```python
from build123d import *

# Parameters (mm, degrees)
SKETCH1_R              = 17.6
BOSS_EXTRUDE1_DEPTH    = 56.8
BOSS_EXTRUDE2_DEPTH    = 4
SKETCH4_R              = 4
SKETCH4_R_2            = 1.5
CUT_EXTRUDE1_DEPTH     = 4
BOSS_EXTRUDE3_DEPTH    = 16
CUT_EXTRUDE2_START     = -14
CUT_EXTRUDE2_OUTLINE_R = 1.45
CUT_EXTRUDE2_DEPTH     = 14
CUT_EXTRUDE3_DEPTH     = 33


# Read off the part's stored shape, not the designer's step: Cut-Extrude2
with BuildPart() as part:
    # Sketch1 → Boss-Extrude1 (new body)
    with BuildSketch(Plane(origin=(0, 0, 0), x_dir=(1, 0, 0), z_dir=(0, 1, 0))):
        with BuildLine():
            Line((-14, -30.7), (-10.2, -30.7))
            ThreePointArc((-10.2, -30.7), (0, -20.5), (10.2, -30.7))
            Line((10.2, -30.7), (14, -30.7))
            add(Edge.make_bspline(
                [(22.4, 0), (22.107939007, -9.890498416), (16.256040946, -13.947885017), (11.388120446, -21.994772931), (14.153535086, -27.339514928), (14, -30.7)],
                knots=[0, 0, 0, 0, 0.589197799, 0.689197799, 1, 1, 1, 1], degree=3))
            ThreePointArc((22.4, 0), (0, 22.4), (-22.4, 0))
            add(Edge.make_bspline(
                [(-22.4, 0), (-22.107939007, -9.890498416), (-16.256040946, -13.947885017), (-11.388120446, -21.994772931), (-14.153535086, -27.339514928), (-14, -30.7)],
                knots=[0, 0, 0, 0, 0.589197799, 0.689197799, 1, 1, 1, 1], degree=3))
        make_face()
        with Locations(Location((0, 0, 0), (0, 0, 270))):
            Circle(SKETCH1_R, mode=Mode.SUBTRACT)
    extrude(amount=BOSS_EXTRUDE1_DEPTH)

    # Sketch3 → Boss-Extrude2 (add)
    with BuildSketch(Plane.XZ):
        with BuildLine():
            ThreePointArc((-14, 30.7), (0, 44.7), (14, 30.7))
            add(Edge.make_bspline(
                [(-14, 30.7), (-12.62265513, 25.007813603), (0.167580012, 13.239499872), (11.954859233, 25.492817672), (14, 30.7)],
                knots=[0, 0, 0, 0, 0.503384006, 1, 1, 1, 1], degree=3))
        make_face()
    extrude(amount=-BOSS_EXTRUDE2_DEPTH)

    # Sketch4 → Cut-Extrude1 (cut)
    with BuildSketch(Plane.XZ):
        with Locations(Location((0, 30.7, 0), (0, 0, 270))):
            Circle(SKETCH4_R)
        with Locations(Location((-7.5, 30.7, 0), (0, 0, 270))):
            Circle(SKETCH4_R_2)
        with Locations(Location((7.5, 30.7, 0), (0, 0, 270))):
            Circle(SKETCH4_R_2)
    extrude(amount=-CUT_EXTRUDE1_DEPTH, mode=Mode.SUBTRACT)

    # Sketch5 → Boss-Extrude3 (add)
    with BuildSketch(Plane(origin=(0, 56.8, 0), x_dir=(1, 0, 0), z_dir=(0, 1, 0))):
        with BuildLine():
            Line((20, 4), (20, -4))
            ThreePointArc((20, -4), (24, 0), (20, 4))
        make_face()
        with BuildLine():
            Line((-20, 4), (-20, -4))
            ThreePointArc((-20, -4), (-24, 0), (-20, 4))
        make_face()
    extrude(amount=-BOSS_EXTRUDE3_DEPTH)

    # Cut-Extrude2 outline → Cut-Extrude2 (cut)
    with BuildSketch(Plane(origin=(0, 56.8, 0), x_dir=(1, 0, 0), z_dir=(0, 1, 0)).offset(CUT_EXTRUDE2_START)):
        with Locations((20, 0)):
            Circle(CUT_EXTRUDE2_OUTLINE_R)
        with Locations((-20, 0)):
            Circle(CUT_EXTRUDE2_OUTLINE_R)
    extrude(amount=CUT_EXTRUDE2_DEPTH, mode=Mode.SUBTRACT)

    # Sketch7 → Cut-Extrude3 (cut)
    with BuildSketch(Plane(origin=(0, 56.8, 0), x_dir=(1, 0, 0), z_dir=(0, 1, 0))):
        with BuildLine():
            Line((-22.083760266, -3.414373025), (-36.083760266, -3.414373025))
            ThreePointArc((-36.083760266, -3.414373025), (0, -36.244940311), (36.083760266, -3.414373025))
            Line((36.083760266, -3.414373025), (22.083760266, -3.414373025))
            ThreePointArc((22.083760266, -3.414373025), (0, -22.346149795), (-22.083760266, -3.414373025))
        make_face()
    extrude(amount=-CUT_EXTRUDE3_DEPTH, mode=Mode.SUBTRACT)


solid = part.part
```
Model file for the job. Use its own axes, mm. A direction names the side the tool comes from. Coordinates: 2 decimals unless noted, no trailing zeros. Loops run counter-clockwise (first coordinate to the right, second up) from the corner with the lowest first, then second, coordinate; pieces in that order, holes last. Notation, with made-up numbers: (-5, 73.25) - (43, 73.25) arc R24 cw to (43, 99.25) - close; hole circle Ø7 at (-30, 84). An arc over 180 degrees is marked (long way). Write item = value, one per line. Start each with the question number.
Item 1: Pull direction Z, two halves, no side cores. Call faces 5 (the face through (23, 40.8, 0)), 6 (the face through (0.493, 28.002, -22.395)), 7 (the face through (-12, 14, 30.7)), 8 (the face through (17.45, 28, -2.29)): +Z half, -Z half, draft (parallel to the pull), parting line (faces both ways), or undercut.
Item 2: Saw through at C-C, the plane y = 47.5. State how many separate pieces and enclosed holes the cut face has, then the cut area to 3 significant figures.
Item 3: Wall check: probe 1 along X at (y, z) = (2, 30); probe 2 along Y at (x, z) = (7.5, 26.5); probe 3 along Z at (x, y) = (-8.5, 29). Give the ranges that are in metal, low to high. Write a range as [from, to].
Item 4: Saw through at D-D, the plane z = 39.5. List the corners of the cut face in (x, y).
Item 5: Saw through at B-B, the plane x = 7.5. List the corners of the cut face in (y, z), then the cut area to 3 significant figures.
Item 6: Drop flat-ended pins along their axis: pin 1 Ø5 at (x, y) = (-3, 26.5) entering from +Z; pin 2 Ø2.5 at (x, z) = (-20, 0) entering from +Y; pin 3 Ø1.9 at (x, y) = (-12, 13) entering from +Z. Give the stop position or say it passes through.
Item 7: 3-axis set-ups, long thin cutter, end or side, ignore diameter. For faces 1 (the face through (-11, 23.8, 24)), 2 (the face through (-20, 42.8, 0)), 3 (the face through (-0.2, 24.2, 20.5)), 4 (the face through (11, 23.8, 24)): which of +Z, -Z, +X, -X, +Y, -Y reach the whole face in a straight line?
Item 8: Saw through at A-A, the plane x = 0. List the corners of the cut face in (y, z).
Answers:
q1.face_5 = draft
q1.face_6 = -Z half
q1.face_7 = +Z half
q1.face_8 = undercut
q2.separate_pieces = 1
q2.enclosed_holes = 3
q2.area = 585 mm2
q3.probe_1 = [-14, -8.83], [-6.17, -3.94], [3.94, 6.17], [8.83, 14]
q3.probe_2 = [0, 4]
q3.probe_3 = [-20.72, -15.41], [15.41, 20.67]
q4.outline = (-10.89, 0) - (10.89, 0) - (10.89, 4) - (-10.89, 4) - close
q5.outline = (0, -21.11) - (56.8, -21.11) - (56.8, -15.92) - (0, -15.92) - close; (0, 15.92) - (56.8, 15.92) - (56.8, 21.05) - (23.8, 21.05) - (23.8, 23.79) - (4, 23.79) - (4, 29.2) - (0, 29.2) - close; (0, 32.2) - (4, 32.2) - (4, 42.52) - (0, 42.52) - close
q5.area = 714 mm2
q6.pin_1 = 21.79
q6.pin_2 = 42.8
q6.pin_3 = 30.7
q7.face_1 = +Z, -X, +Y
q7.face_2 = +Y
q7.face_3 = +Z, +Y
q7.face_4 = +Z, +X, +Y
q8.outline = (0, -22.4) - (56.8, -22.4) - (56.8, -17.6) - (0, -17.6) - close; (0, 17.6) - (56.8, 17.6) - (56.8, 20.5) - (4, 20.5) - (4, 26.7) - (0, 26.7) - close; (0, 34.7) - (4, 34.7) - (4, 44.7) - (0, 44.7) - close
